Read the model definition and answer for the solid it produces. Units are mm, in the model's axes. A direction names the side the tool comes from. Give positions to 0.01 mm unless a question says otherwise; leave off trailing zeros. Write each loop counter-clockwise with the first axis right and the second up, starting at its lowest first coordinate (ties: lowest second). Pieces come first, ordered by that corner, then holes. Notation, with made-up numbers: (22.5, 34.25) -> (36.5, 34.25) arc R31 ccw to (36.5, 63.25) -> close; hole circle Ø1 at (-12, -32). An arc over 180 degrees is marked (long way). Use a Markdown table: item, result.
from build123d import *

# Parameters (mm, degrees)
BOSS_EXTRU_1_DEPTH = 25
ESQUISSE2_R        = 3
BOSS_EXTRU_2_DEPTH = 2
ESQUISSE3_R        = 1
BOSS_EXTRU_3_DEPTH = 8


with BuildPart() as part:
    # Esquisse1 → Boss.-Extru.1 (new body)
    with BuildSketch(Plane.XY):
        with BuildLine():
            Line((-6.614378278, 7.5), (6.614378278, 7.5))
            ThreePointArc((6.614378278, 7.5), (10, 0), (6.614378278, -7.5))
            Line((6.614378278, -7.5), (-6.614378278, -7.5))
            ThreePointArc((-6.614378278, -7.5), (-10, 0), (-6.614378278, 7.5))
        make_face()
    extrude(amount=BOSS_EXTRU_1_DEPTH)

    # Esquisse2 → Boss.-Extru.2 (add)
    with BuildSketch(Plane.XY.offset(25)):
        Circle(ESQUISSE2_R)
    extrude(amount=BOSS_EXTRU_2_DEPTH)

    # Esquisse3 → Boss.-Extru.3 (add)
    with BuildSketch(Plane.XY.offset(27)):
        Circle(ESQUISSE3_R)
    extrude(amount=BOSS_EXTRU_3_DEPTH)


solid = part.part
Item 1: A cutting plane is placed at D-D (x = 3.5). Give the vertices of the cut face in (y, z), then the cut area to 3 significant figures.
Return value:
| item | result |
|---|---|
| outline | (-7.5, 0) -> (7.5, 0) -> (7.5, 25) -> (-7.5, 25) -> close |
| area | 375 mm^2 |
Item 2: A tool of negligible diameter and unlimited length cuts with its end or side. For faces 1 (the face through (10, 0, 12)), 2 (the face through (0.1, 3.4, 25)), from which of +Z, -Z, +X, -X, +Y, -Y can it reach the whole face along a straight path? Write none if from no direction.
Return value:
| item | result |
|---|---|
| face 1 | +Z, -Z, +X |
| face 2 | +Z |
Item 3: A cutting plane is placed at A-A (y = 0). Give the vertices of the cut face in (x, z).
Return value:
| item | result |
|---|---|
| outline | (-10, 0) -> (10, 0) -> (10, 25) -> (3, 25) -> (3, 27) -> (1, 27) -> (1, 35) -> (-1, 35) -> (-1, 27) -> (-3, 27) -> (-3, 25) -> (-10, 25) -> close |
Item 4: A cutting plane is placed at C-C (z = 11.5). Give the vertices of the cut face in (x, y), then the cut area to 3 significant figures.
Return value:
| item | result |
|---|---|
| outline | (-6.61, -7.5) -> (6.61, -7.5) arc R10 ccw to (6.61, 7.5) -> (-6.61, 7.5) arc R10 ccw to start |
| area | 269 mm^2 |
Item 5: A cutting plane is placed at B-B (x = 0). Give the vertices of the cut face in (y, z), then the cut area to 3 significant figures.
Return value:
| item | result |
|---|---|
| outline | (-7.5, 0) -> (7.5, 0) -> (7.5, 25) -> (3, 25) -> (3, 27) -> (1, 27) -> (1, 35) -> (-1, 35) -> (-1, 27) -> (-3, 27) -> (-3, 25) -> (-7.5, 25) -> close |
| area | 403 mm^2 |
Item 6: Each of these flat-tipped pins is pushed along its axis until it touches: P1, Ø1.5, axis at y = 2.5, z = 16, coming from the -X side; P2, Ø1, axis at x = -7.5, z = 22, coming from the -Y side; P3, Ø1, axis at y = -2, z = 21, coming from the +X side; P4, Ø1.5, axis at x = -2.5, z = 30.5, coming from the +Y side. Where does it stop, or does it pass through?
Return value:
| item | result |
|---|---|
| P1 | x = -9.85 |
| P2 | y = -7.14 |
| P3 | x = 9.89 |
| P4 | through |
Item 7: Straight lines are drawn through the part: line 1 along Z through (x, y) = (-1, 2.5); line 2 along Z through (x, y) = (-6, -5.5); line 3 along X through (y, z) = (2, 17). For each, find the intervals that lie inside material, in ascending order. Write a range as [from, to].
Return value:
| item | result |
|---|---|
| line 1 | [0, 27] |
| line 2 | [0, 25] |
| line 3 | [-9.8, 9.8] |
